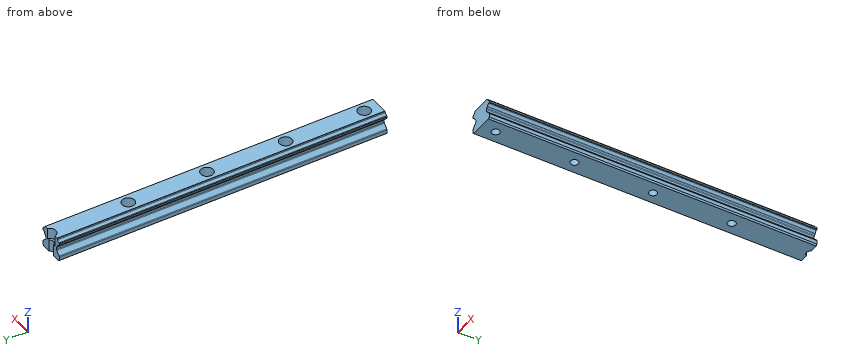
Autodesk Inventor part; units mm, degrees
ref_plane "YZ Plane" through (0, 0, 0) normal (1, 0, 0) x (0, 1, 0)
ref_plane "XZ Plane" through (0, 0, 0) normal (0, 1, 0) x (-1, 0, 0)
ref_plane "XY Plane" through (0, 0, 0) normal (0, 0, 1) x (1, 0, 0)
sketch "Sketch1" plane through (0, 0, 0) normal (0, 1, 0) x (-1, 0, 0)
  arc A0 (-6.7759, -1.5867) -> (-6.483, -0.8796) centre (-7.483, -0.8796) ccw
  line L0 (-7.1187, 8.7305) -> (7.3527, 8.7305)
  line L1 (9.117, -8.7695) -> (-8.883, -8.7695)
  line L2 (6.717, 0.6806) -> (6.717, -0.8796)
  arc A1 (7.0099, 1.3877) -> (6.717, 0.6806) centre (7.717, 0.6806) ccw
  line L3 (7.7471, 2.1249) -> (7.0099, 1.3877)
  arc A2 (6.717, -0.8796) -> (7.0099, -1.5867) centre (7.717, -0.8796) ccw
  arc A3 (-9.5901, -4.4009) -> (-9.883, -5.108) centre (-8.883, -5.108) ccw
  line L4 (-9.883, -7.7695) -> (-9.883, -5.108)
  line L5 (-8.883, -8.7695) -> (-9.883, -7.7695)
  line L6 (-9.5901, -4.4009) -> (-6.7759, -1.5867)
  line L7 (10.117, 5.7591) -> (10.117, 4.7019)
  arc A4 (10.117, 5.7591) -> (9.9705, 6.1127) centre (9.617, 5.7591) ccw
  line L8 (9.8076, 6.2756) -> (9.9705, 6.1127)
  arc A5 (9.8076, 6.2756) -> (9.5394, 6.4246) centre (9.4424, 5.9341) ccw
  arc A6 (7.9651, 7.9985) -> (9.5394, 6.4246) centre (9.9271, 8.3866) ccw
  arc A7 (7.9651, 7.9985) -> (7.7495, 8.3337) centre (7.4717, 7.918) ccw
  line L9 (7.3527, 8.7305) -> (7.7495, 8.3337)
  line L10 (-6.483, -0.8796) -> (-6.483, 0.6806)
  arc A8 (-6.483, 0.6806) -> (-6.7759, 1.3877) centre (-7.483, 0.6806) ccw
  line L11 (-6.7759, 1.3877) -> (-7.5132, 2.1249)
  arc A9 (-7.7298, 2.463) -> (-7.5132, 2.1249) centre (-7.2359, 2.541) ccw
  arc A10 (-7.7298, 2.463) -> (-9.3148, 4.048) centre (-9.6936, 2.0842) ccw
  line L12 (-9.5736, 4.1854) -> (-9.7366, 4.3483)
  arc A11 (-9.883, 4.7019) -> (-9.7366, 4.3483) centre (-9.383, 4.7019) ccw
  line L13 (-9.883, 4.7019) -> (-9.883, 5.7591)
  arc A12 (-9.7366, 6.1127) -> (-9.883, 5.7591) centre (-9.383, 5.7591) ccw
  arc A13 (9.9705, 4.3483) -> (10.117, 4.7019) centre (9.617, 4.7019) ccw
  line L14 (9.9705, 4.3483) -> (9.8076, 4.1854)
  arc A14 (9.5488, 4.048) -> (9.8076, 4.1854) centre (9.4541, 4.539) ccw
  arc A15 (9.5488, 4.048) -> (7.9638, 2.463) centre (9.9276, 2.0842) ccw
  arc A16 (7.7471, 2.1249) -> (7.9638, 2.463) centre (7.4699, 2.541) ccw
  line L15 (7.0099, -1.5867) -> (9.8241, -4.4009)
  arc A17 (10.117, -5.108) -> (9.8241, -4.4009) centre (9.117, -5.108) ccw
  line L16 (10.117, -5.108) -> (10.117, -7.7695)
  line L17 (10.117, -7.7695) -> (9.117, -8.7695)
  line L18 (-9.7366, 6.1127) -> (-9.5736, 6.2756)
  arc A18 (-9.3054, 6.4246) -> (-9.5736, 6.2756) centre (-9.2085, 5.9341) ccw
  arc A19 (-9.3054, 6.4246) -> (-7.7312, 7.9985) centre (-9.6932, 8.3866) ccw
  arc A20 (-7.5156, 8.3337) -> (-7.7312, 7.9985) centre (-7.2377, 7.918) ccw
  line L19 (-7.5156, 8.3337) -> (-7.1187, 8.7305)
  arc A21 (-9.5736, 4.1854) -> (-9.3148, 4.048) centre (-9.2201, 4.539) ccw
  point P0 (0, 0)
  point P1 (0.117, -0.039)
  point P2 (0.117, 5.2305)
extrude "Extrusion1" add sketch "Sketch1" along normal blind 250
sketch "Sketch2" plane through (-7.3527, 0, 8.7305) normal (0, 0, 1) x (1, 0, 0)
  circle A0 centre (7.2357, 11.1125) radius 3
  line L0 (0, 0) -> (14.4714, 0)
  line L1 (-2.7643, 0) -> (-2.7643, 250)
  line L2 (17.2357, 0) -> (17.2357, 250)
  circle A1 centre (7.2357, 71.1125) radius 3
  circle A2 centre (7.2357, 131.1125) radius 3
  circle A3 centre (7.2357, 191.1125) radius 3
  circle A4 centre (7.2357, 251.1125) radius 3
  point P0 (7.3527, 0)
  dimension "d2" = 6
  dimension "d3" = 11.1125
  dimension "d4" = 20
  dimension "d5" = 10
  dimension "d8" = 60
  dimension "d18" = 60
extrude "Extrusion2" cut sketch "Sketch2" against normal through all contours A0 | A1 | A2 | A3
sketch "Sketch3" plane through (-7.3527, 0, 8.7305) normal (0, 0, 1) x (1, 0, 0)
  circle A0 centre (7.2357, 71.1125) radius 3
  circle A1 centre (7.2357, 131.1125) radius 3
  circle A2 centre (7.2357, 11.1125) radius 3
  circle A3 centre (7.2357, 191.1125) radius 3
  line L0 (0, 0) -> (14.4714, 0)
  line L1 (14.4714, 0) -> (14.4714, 250)
  line L2 (0, 250) -> (14.4714, 250)
  line L3 (0, 0) -> (0, 250)
  circle A4 centre (7.2357, 11.1125) radius 4.75
  circle A5 centre (7.2357, 71.1125) radius 4.75
  circle A6 centre (7.2357, 131.1125) radius 4.75
  circle A7 centre (7.2357, 191.1125) radius 4.75
  circle A8 centre (7.2357, 251.1125) radius 4.75
  point P0 (7.3527, 0)
  point P1 (11.8536, 250)
  point P2 (2.6178, 250)
  dimension "d15" = 9.5
  dimension "d21" = 60
extrude "Extrusion3" cut sketch "Sketch3" against normal blind 8.4 contours A4 | A5 | A6 | A7
extrude "Extrusion4" cut sketch "Sketch2" against normal through all contours A4
extrude "Extrusion5" cut sketch "Sketch3" against normal up to surface (8.4 mm away) contours L2 A8 picked at (8.3547, 248.0358)
equation "\"d5\" = 0.5 * d4"
properties part number "HGR20R-LinearRail200mm" material "Stainless Steel"
Design review of the part built by this model. Coordinates are the model's own, in mm. Round coordinates to 2 decimals unless told otherwise and drop trailing zeros. One line per item, written item: value. Start each with the question number.
1) To check wall thickness, follow L1, parallel to Y at x = -3, z = 7; L2, parallel to Y at x = 3, z = 7; L3, parallel to X at y = 117.5, z = -5. State the ranges of each line that lie inside material, in increasing order. Write a range as from..to.
2) Consider section A-A on x = 0. Give the number of separate pieces and of enclosed holes in the cut face, then the cut area to 3 significant figures.
3) Insertion check: pin 1 Ø1.2 at (y, z) = (142, -0.5) entering from +X; pin 2 Ø1.1 at (x, y) = (0, 248.5) entering from +Z; pin 3 Ø0.5 at (y, z) = (99.5, 0) entering from -X. Each pin has a flat end and moves straight along its axis. Give the tip position at first contact, or say it passes through.
Reported:
1. L1: y = 0..7.34, 14.89..67.34, 74.89..127.34, 134.89..187.34, 194.89..247.34
1. L2: y = 0..7.53, 14.7..67.53, 74.7..127.53, 134.7..187.53, 194.7..247.53
1. L3: x = -10.11..9.88
2. separate pieces: 5
2. enclosed holes: 0
2. area: 3,790 mm^2
3. pin 1: stops at x = 6.51
3. pin 2: stops at z = 0.33
3. pin 3: stops at x = -6.72
